from build123d import *

# Parameters (mm, degrees)
F2_DEPTH = 10.16
F1_R     = 9.1481918334
F1_R_2   = 9.4297469702
F1_R_3   = 11.4352472888
F3_DEPTH = 15.24
F4_R     = 8.7387989597
F4_R_2   = 8.7387973247
F4_R_3   = 11.4352472888
F5_DEPTH = 5.08


with BuildPart() as f2:
    # F0 (on Top) → F2 (new body)
    with BuildSketch(Plane.XY):
        with BuildLine():
            ThreePointArc((22.3403535783, -72.851551816), (61.2730566508, -45.2995864072), (76.2, 0))
            ThreePointArc((76.2, 0), (74.7105977036, 14.9922176738), (70.3006144153, 29.3983607168))
            Line((70.3006144153, 29.3983607168), (22.3403535783, 9.3423048788))
            Line((22.3403535783, 9.3423048788), (22.3403535783, -72.851551816))
        make_face()
        with BuildLine():
            Line((22.3403535783, 9.3423048788), (70.3006144153, 29.3983607168))
            ThreePointArc((70.3006144153, 29.3983607168), (64.0396717964, 41.2960099309), (55.785185421, 51.9081215952))
            Line((55.785185421, 51.9081215952), (21.8996389933, 37.3568432093))
            Line((21.8996389933, 37.3568432093), (22.3403535783, 37.3568432093))
            Line((22.3403535783, 37.3568432093), (22.3403535783, 9.3423048788))
        make_face()
        with BuildLine():
            ThreePointArc((55.785185421, 51.9081215952), (64.0396717964, 41.2960099309), (70.3006144153, 29.3983607168))
            Line((70.3006144153, 29.3983607168), (210.9018432458, 88.1950821504))
            Line((210.9018432458, 88.1950821504), (210.9018432458, 118.5189898936))
            Line((210.9018432458, 118.5189898936), (55.785185421, 51.9081215952))
        make_face()
        with BuildLine():
            Line((22.3403535783, -191.2431567907), (22.3403535783, -72.851551816))
            ThreePointArc((22.3403535783, -72.851551816), (9.7794429224, -75.5698517673), (-3.0596464217, -76.1385484743))
            Line((-3.0596464217, -76.1385484743), (-3.0596464217, -191.2431567907))
            Line((-3.0596464217, -191.2431567907), (22.3403535783, -191.2431567907))
        make_face()
        with BuildLine():
            ThreePointArc((-3.0596464217, -76.1385484743), (9.7794429224, -75.5698517673), (22.3403535783, -72.851551816))
            Line((22.3403535783, -72.851551816), (22.3403535783, 9.3423048788))
            Line((22.3403535783, 9.3423048788), (0, 0))
            Line((0, 0), (-3.0596464217, 1.4057470004))
            Line((-3.0596464217, 1.4057470004), (-3.0596464217, -76.1385484743))
        make_face()
        with BuildLine():
            Line((21.8996389933, 37.3568432093), (55.785185421, 51.9081215952))
            ThreePointArc((55.785185421, 51.9081215952), (0.8041557349, 76.1957566637), (-54.6772246178, 53.0739211675))
            Line((-54.6772246178, 53.0739211675), (-3.0596464217, 29.3583522044))
            Line((-3.0596464217, 29.3583522044), (-3.0596464217, 37.3568432093))
            Line((-3.0596464217, 37.3568432093), (21.8996389933, 37.3568432093))
        make_face()
        with BuildLine():
            ThreePointArc((-69.2414887941, 31.8128312096), (-64.9633637698, -39.8271436047), (-3.0596464217, -76.1385484743))
            Line((-3.0596464217, -76.1385484743), (-3.0596464217, 1.4057470004))
            Line((-3.0596464217, 1.4057470004), (-69.2414887941, 31.8128312096))
        make_face()
        with BuildLine():
            Line((-3.0596464217, 29.3583522044), (-54.6772246178, 53.0739211675))
            ThreePointArc((-54.6772246178, 53.0739211675), (-62.8646989173, 43.0635533837), (-69.2414887941, 31.8128312096))
            Line((-69.2414887941, 31.8128312096), (-3.0596464217, 1.4057470004))
            Line((-3.0596464217, 1.4057470004), (-3.0596464217, 29.3583522044))
        make_face()
        with BuildLine():
            ThreePointArc((-69.2414887941, 31.8128312096), (-62.8646989173, 43.0635533837), (-54.6772246178, 53.0739211675))
            Line((-54.6772246178, 53.0739211675), (-197.1201893125, 118.5189898936))
            Line((-197.1201893125, 118.5189898936), (-207.7244663824, 95.4384936289))
            Line((-207.7244663824, 95.4384936289), (-69.2414887941, 31.8128312096))
        make_face()
        Polygon((0, 0), (22.3403535783, 9.3423048788), (22.3403535783, 37.3568432093), (21.8996389933, 37.3568432093), (0, 27.952605204), (-3.0596464217, 29.3583522044), (-3.0596464217, 1.4057470004), align=None)
        Polygon((0, 27.952605204), (21.8996389933, 37.3568432093), (-3.0596464217, 37.3568432093), (-3.0596464217, 29.3583522044), align=None)
    extrude(amount=F2_DEPTH)

    # F1 (on Top) → F3 (join)
    with BuildSketch(Plane.XY):
        with Locations((-187.970161438, 101.8863245845)):
            Circle(F1_R)
        with Locations((9.4301495701, -176.3151586056)):
            Circle(F1_R_2)
        with Locations((193.1931376457, 95.4085886478)):
            Circle(F1_R_3)
    extrude(amount=F3_DEPTH)

    # F4 (on Top) → F5 (join)
    with BuildSketch(Plane.XY):
        with Locations((9.941550903, -177.6788830757)):
            Circle(F4_R)
        with Locations((-191.5499567986, 102.5681942701)):
            Circle(F4_R_2)
        with Locations((195.068269968, 96.431389451)):
            Circle(F4_R_3)
    extrude(amount=-F5_DEPTH)


solid = f2.part
Read the model definition and answer for the solid it produces. Units are mm, in the model's axes. A direction names the side the tool comes from. Give positions to 0.01 mm unless a question says otherwise; leave off trailing zeros. Write each loop counter-clockwise with the first axis right and the second up, starting at its lowest first coordinate (ties: lowest second). Pieces come first, ordered by that corner, then holes. Notation, with made-up numbers: (-36.5, 52) -> (-15.5, 52) arc R7 cw to (-15.5, 65) -> close; hole circle Ø4 at (10, 10). An arc over 180 degrees is marked (long way). Answer as a JSON object with one key per item and string values. Group by question number.
1) Find section D-D (y = -60). Write down the section's boundary in (x, z).
2) Consider L1, parallel to X at y = -126.5, z = 3.75; L2, parallel to Z at x = 180.5, y = 102; L3, parallel to X at y = 103.5, z = -2.75. Determine where each line is inside the solid, lowest interval first. Write a range as from..to.
3) A tool of negligible diameter and unlimited length cuts with its end or side. For faces 1 (the flat face through (134.43, 85.68, 5.01)), 2 (the flat face through (-3.06, -133, 5)), 3 (the cylindrical face through (192.589, 85.268, -2.504)), 4 (the cylindrical face through (7.39, -185.52, 12.66)), from which of +Z, -Z, +X, -X, +Y, -Y can it reach the whole face along a straight path? Write none if from no direction.
4) Find section A-A (z = 5). Write down the section's boundary in (x, y), and give its area (3 significant figures).
5) Each of these flat-tipped pins is pushed along its axis until it touches: P1, Ø8, axis at x = 104, z = 12, coming from the -Y side; P2, Ø6, axis at x = 106.5, z = 7, coming from the +Y side; P3, Ø1.5, axis at x = 76, y = 53.5, coming from the -Z side; P4, Ø8, axis at x = 12.5, z = 11.5, coming from the -Y side. Where does it stop, or does it pass through?
6) Find section B-B (y = -123.5). Write down the section's boundary in (x, z), and give its area (3 significant figures).
7) Find section C-C (x = 14.5). Write down the section's boundary in (y, z), and give its area (3 significant figures).
8) The mould has two halves that part along Y. Classify faces 5 (the cylindrical face through (13.974, -185.432, -2.504)), 6 (the cylindrical face through (-65.504, -38.932, 5.009)), 7 (the flat face through (22.34, -133, 5)): +Y half, -Y half, draft (parallel to the pull), parting line (faces both ways), or undercut.
Values follow:
{
 "1": {"outline": "(-46.97, 0) -> (46.97, 0) -> (46.97, 10.16) -> (-46.97, 10.16) -> close"},
 "2": {"L1": "x = -3.06..22.34", "L2": "z = 0..10.16", "L3": "x = -200.24..-182.86, 186.08..204.06"},
 "3": {"face 1": "+Z, -Z, +Y", "face 2": "+Z, -Z, -X, -Y", "face 3": "-Z", "face 4": "+Z"},
 "4": {"outline": "(-207.72, 95.44) -> (-69.24, 31.81) arc R76.2 ccw to (-3.06, -76.14) -> (-3.06, -191.24) -> (22.34, -191.24) -> (22.34, -72.85) arc R76.2 ccw to (70.3, 29.4) -> (210.9, 88.2) -> (210.9, 118.52) -> (55.79, 51.91) arc R76.2 ccw to (-54.68, 53.07) -> (-197.12, 118.52) -> close", "area": "29,400 mm2"},
 "5": {"P1": "stops at y = 42.01", "P2": "stops at y = 74.97", "P3": "stops at z = 0", "P4": "stops at y = -191.24"},
 "6": {"outline": "(-3.06, 0) -> (22.34, 0) -> (22.34, 10.16) -> (-3.06, 10.16) -> close", "area": "258 mm2"},
 "7": {"outline": "(-191.24, 0) -> (-185.13, 0) -> (-185.13, -5.08) -> (-170.22, -5.08) -> (-170.22, 0) -> (74.81, 0) -> (74.81, 10.16) -> (-168.36, 10.16) -> (-168.36, 15.24) -> (-184.27, 15.24) -> (-184.27, 10.16) -> (-191.24, 10.16) -> close", "area": "2,860 mm2"},
 "8": {"face 5": "parting line", "face 6": "undercut", "face 7": "draft"}
}
